Source: CAD feature listing. Evaluate the final solid. Frame: model axes, mm. Face numbers are marked on the shaded views. A direction names the side the tool comes from. Round coordinates to 2 decimals unless told otherwise and drop trailing zeros. Write each loop counter-clockwise with the first axis right and the second up, starting at its lowest first coordinate (ties: lowest second). Pieces come first, ordered by that corner, then holes.
```python
from build123d import *

# Parameters (mm, degrees)
ESQUISSE3_R        = 20
ESQUISSE3_R_2      = 1.5
ESQUISSE3_W        = 6.1
ESQUISSE3_H        = 6.1
BOSS_EXTRU_2_DEPTH = 1.58
ESQUISSE5_W        = 6.1
ESQUISSE5_H        = 6.1
BOSS_EXTRU_3_DEPTH = 5.2
ESQUISSE6_R        = 1.8
BOSS_EXTRU_4_DEPTH = 3.6
ESQUISSE7_W        = 8.59
ESQUISSE7_H        = 20.3
BOSS_EXTRU_5_DEPTH = 9.92


with BuildPart() as part:
    # Esquisse3 → Boss.-Extru.2 (new body)
    with BuildSketch(Plane.XY):
        Circle(ESQUISSE3_R)
        with Locations((-12.5, -10)):
            Circle(ESQUISSE3_R_2, mode=Mode.SUBTRACT)
        with Locations((12.5, -10)):
            Circle(ESQUISSE3_R_2, mode=Mode.SUBTRACT)
        with Locations((12.5, 10)):
            Circle(ESQUISSE3_R_2, mode=Mode.SUBTRACT)
        with Locations((-15, 0)):
            Rectangle(ESQUISSE3_W, ESQUISSE3_H, mode=Mode.SUBTRACT)
        with Locations((15, 0)):
            Rectangle(ESQUISSE3_W, ESQUISSE3_H, mode=Mode.SUBTRACT)
        with Locations((0, 15)):
            Rectangle(ESQUISSE3_W, ESQUISSE3_H, mode=Mode.SUBTRACT)
        with Locations((0, -15)):
            Rectangle(ESQUISSE3_W, ESQUISSE3_H, mode=Mode.SUBTRACT)
        Rectangle(ESQUISSE3_W, ESQUISSE3_H, mode=Mode.SUBTRACT)
    extrude(amount=BOSS_EXTRU_2_DEPTH)

    # Esquisse5 → Boss.-Extru.3 (add)
    with BuildSketch(Plane(origin=(0, 0, 0), x_dir=(-1, 0, 0), z_dir=(0, 0, -1))):
        with Locations((0, 15)):
            Rectangle(ESQUISSE5_W, ESQUISSE5_H)
        with Locations((-15, 0)):
            Rectangle(ESQUISSE5_W, ESQUISSE5_H)
        with Locations((15, 0)):
            Rectangle(ESQUISSE5_W, ESQUISSE5_H)
        Rectangle(ESQUISSE5_W, ESQUISSE5_H)
        with Locations((0, -15)):
            Rectangle(ESQUISSE5_W, ESQUISSE5_H)
    extrude(amount=-BOSS_EXTRU_3_DEPTH)

    # Esquisse6 → Boss.-Extru.4 (add)
    with BuildSketch(Plane.XY.offset(5.2)):
        Circle(ESQUISSE6_R)
        with Locations((0, 15)):
            Circle(ESQUISSE6_R)
        with Locations((15, 0)):
            Circle(ESQUISSE6_R)
        with Locations((0, -15)):
            Circle(ESQUISSE6_R)
        with Locations((-15, 0)):
            Circle(ESQUISSE6_R)
    extrude(amount=BOSS_EXTRU_4_DEPTH)

    # Esquisse7 → Boss.-Extru.5 (add)
    with BuildSketch(Plane.XY):
        with Locations((-6.715, 0.63)):
            Rectangle(ESQUISSE7_W, ESQUISSE7_H)
    extrude(amount=-BOSS_EXTRU_5_DEPTH)


solid = part.part
```
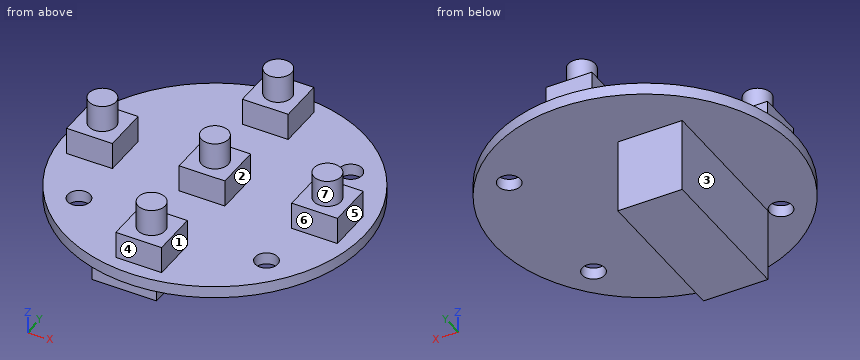
Q1. Section query C-C, the plane x = 12.5. Output: boundary loops of the cut face in (y, z).
Q2. Set-up query: the marked faces 1, 2, 3 and 4. Return all of +Z, -Z, +X, -X, +Y, -Y with unobstructed straight access to the full face (end or side cutting, diameter ignored); none if empty.
Q3. Pin query (flat end, axial travel): P1, Ø1.8, axis at x = -13.5, z = 4, coming from the -Y side; P2, Ø4, axis at x = -15, z = -4.5, coming from the +Y side; P3, Ø3, axis at x = 0.5, z = 4, coming from the -Y side; P4, Ø8, axis at x = -11, z = 1, coming from the -Y side (3 decimals). Return the tip coordinate at first contact, or that it passes through.
Q4. Section query D-D, the plane z = 0.5. Output: boundary loops of the cut face in (x, y), and give its area (3 significant figures).
Q5. Line query: line 1 (Y direction, x = -1.5, z = 5.75); line 2 (X direction, y = -1, z = 7); line 3 (Z direction, x = 10, y = -5). Output: solid intervals per line, ascending.
Q6. Mould query, pull axis X, two halves, no side actions, for the marked faces 5, 6 and 7. Classes: pulls with the +X half, pulls with the -X half, needs draft (parallel to the pull), parting line crosses it, or undercut.
Q7. Section query A-A, the plane z = 6.25. Output: boundary loops of the cut face in (x, y), and give its area (3 significant figures).
Q8. Section query B-B, the plane y = -10.5. Output: boundary loops of the cut face in (x, z), and give its area (3 significant figures).
Filled in:
1. outline: (-15.61, 0) - (-11.5, 0) - (-11.5, 1.58) - (-15.61, 1.58) - close; (-8.5, 0) - (8.5, 0) - (8.5, 1.58) - (3.05, 1.58) - (3.05, 5.2) - (-3.05, 5.2) - (-3.05, 1.58) - (-8.5, 1.58) - close; (11.5, 0) - (15.61, 0) - (15.61, 1.58) - (11.5, 1.58) - close
2. face 1: +Z, +X, +Y, -Y
2. face 2: +Z, +Y, -Y
2. face 3: -Z, -X, +Y, -Y
2. face 4: +Z, +X, -X, -Y
3. P1: stops at y = -3.05
3. P2: passes through
3. P3: stops at y = -18.05
3. P4: stops at y = -18.735
4. outline: circle Ø40 at (0, 0); hole circle Ø3 at (-12.5, -10); hole circle Ø3 at (12.5, -10); hole circle Ø3 at (12.5, 10)
4. area: 1,240 mm2
5. line 1: y = -15.99 to -14.01, -0.99 to 0.99, 14.01 to 15.99
5. line 2: x = -16.5 to -13.5, -1.5 to 1.5, 13.5 to 16.5
5. line 3: z = 0 to 1.58
6. face 5: pulls with the +X half
6. face 6: needs draft
6. face 7: undercut
7. outline: circle Ø3.6 at (-15, 0); circle Ø3.6 at (0, -15); circle Ø3.6 at (0, 0); circle Ø3.6 at (0, 15); circle Ø3.6 at (15, 0)
7. area: 50.9 mm2
8. outline: (-17.02, 0) - (-13.91, 0) - (-13.91, 1.58) - (-17.02, 1.58) - close; (-11.09, 0) - (11.09, 0) - (11.09, 1.58) - (-11.09, 1.58) - close; (13.91, 0) - (17.02, 0) - (17.02, 1.58) - (13.91, 1.58) - close
8. area: 44.9 mm2
